Part print with two shaded views. Sizes in mm from the minimum x, y, z corner. Round coordinates to 2 decimals unless told otherwise and drop trailing zeros. Order: outer loops, then holes, each group sorted by start corner. A loop starts at its lowest first (then second) coordinate and runs counter-clockwise, first axis right, second up. Notation, with made-up numbers: M 80.5,35 L 131.5,35 A24 ccw 131.5,58 Z; hole C 52,-27 d9. An arc over 180 degrees is marked long. Answer as a JSON object with one key per item and string values.
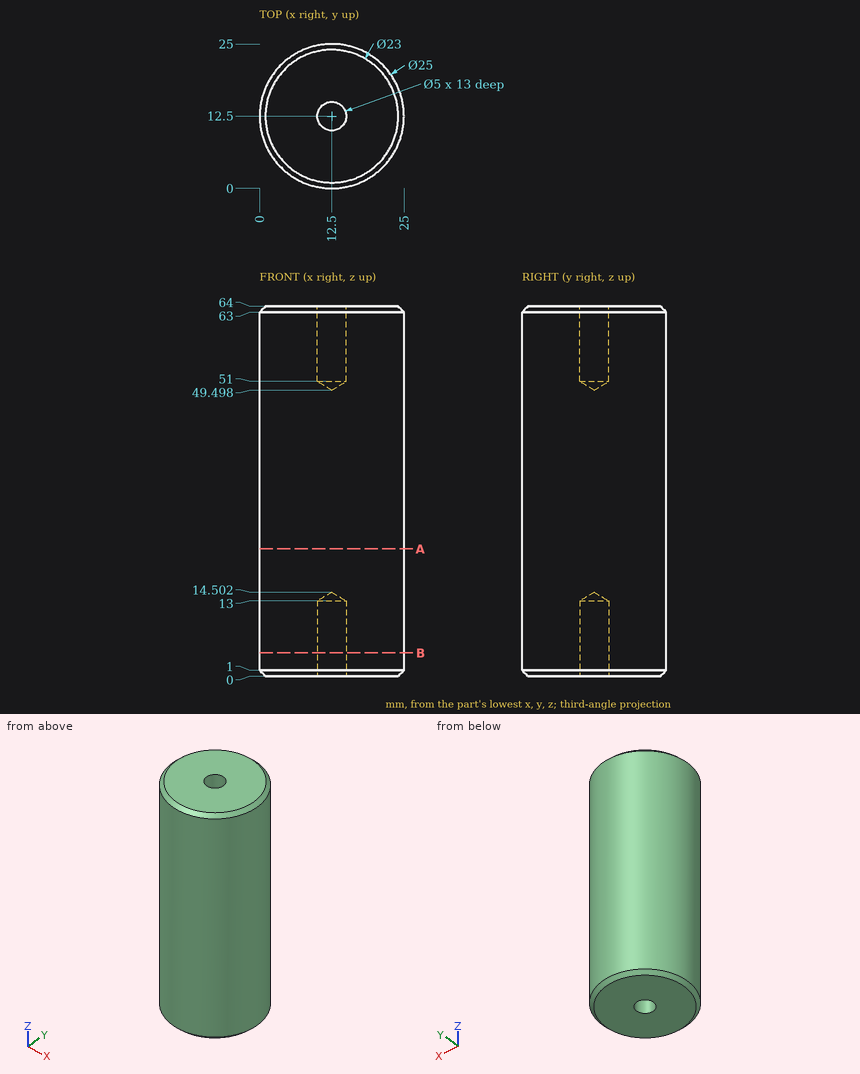
Item 1: Saw through at A-A on z = 22. List the corners of the cut face in (x, y), and give its area (3 significant figures).
Worked answers:
{"outline": "C 12.5,12.5 d25", "area": "491 mm2"}
Item 2: Wall check: line 1 along Y through (x, z) = (12.5, 10.75); line 2 along Y through (x, z) = (11.5, 7.5); line 3 along Y through (x, z) = (8, 5). Give the ranges that are in metal, low to high. Write a range as [from, to].
Worked answers:
{"line 1": "y = [0, 10], [15, 25]", "line 2": "y = [0.04, 10.21], [14.79, 24.96]", "line 3": "y = [0.84, 24.16]"}
Item 3: Saw through at B-B on z = 4. List the corners of the cut face in (x, y).
Worked answers:
{"outline": "C 12.5,12.5 d25; hole C 12.5,12.5 d5"}
Item 4: Drop flat-ended pins along their axis: pin 1 Ø8 at (x, y) = (9, 4) entering from -Z; pin 2 Ø5 at (y, z) = (20.5, 50.5) entering from +X (3 decimals); pin 3 Ø1.5 at (x, z) = (17.5, 51.5) entering from +Y (1 decimal); pin 4 Ø6 at (y, z) = (8.5, 9) entering from -X. Give the stop position or say it passes through.
Worked answers:
{"pin 1": "stops at z = 0", "pin 2": "stops at x = 23.725", "pin 3": "stops at y = 24.3", "pin 4": "stops at x = 0.04"}
